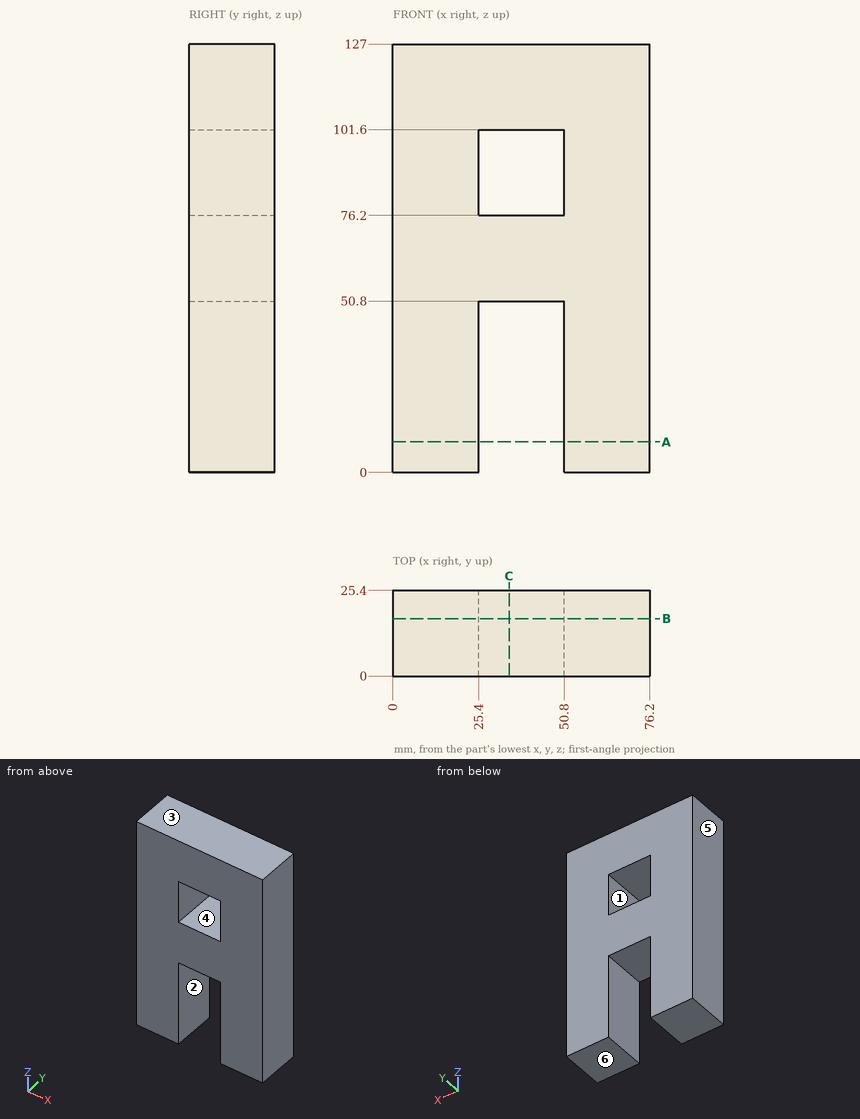
Part print with two shaded views. Sizes in mm from the minimum x, y, z corner. A direction names the side the tool comes from. Give positions to 0.01 mm unless a question says otherwise; leave off trailing zeros. Order: outer loops, then holes, each group sorted by start corner. A loop starts at its lowest first (then second) coordinate and runs counter-clockwise, first axis right, second up. Notation, with made-up numbers: M -12.5,0.5 L 13.5,0.5 A20 ccw 13.5,33.5 Z; hole C -11,42 d8. An arc over 180 degrees is marked long. Put each result on its own line as item: value.
Item 1: Cut at C-C on x = 34.5. Write the cut outline in (y, z), then the cut area to 3 significant figures.
Results are:
outline: M 0,50.8 L 25.4,50.8 L 25.4,76.2 L 0,76.2 Z; M 0,101.6 L 25.4,101.6 L 25.4,127 L 0,127 Z
area: 1,290 mm2
Item 2: Cut at B-B on y = 17. Write the cut outline in (x, z).
Results are:
outline: M 0,0 L 25.4,0 L 25.4,50.8 L 50.8,50.8 L 50.8,0 L 76.2,0 L 76.2,127 L 0,127 Z; hole M 25.4,76.2 L 50.8,76.2 L 50.8,101.6 L 25.4,101.6 Z
Item 3: Pull direction Z, two halves, no side cores. Call the marked faces 4, 5 and 6: +Z half, -Z half, draft (parallel to the pull), parting line (faces both ways), or undercut.
Results are:
face 4: undercut
face 5: draft
face 6: -Z half
Item 4: Cut at A-A on z = 9. Write the cut outline in (x, y), then the cut area to 3 significant figures.
Results are:
outline: M 0,0 L 25.4,0 L 25.4,25.4 L 0,25.4 Z; M 50.8,0 L 76.2,0 L 76.2,25.4 L 50.8,25.4 Z
area: 1,290 mm2
Item 5: Drop flat-ended pins along their axis: pin 1 Ø12 at (x, z) = (39.5, 95) entering from -Y; pin 2 Ø7.5 at (y, z) = (7.5, 85) entering from -X; pin 3 Ø5 at (x, y) = (34.5, 18.5) entering from -Z. Give the stop position or say it passes through.
Results are:
pin 1: through
pin 2: x = 0
pin 3: z = 50.8
Item 6: Which spindle directions (+Z, -Z, +X, -X, +Y, -Y) get a long thin tool onto all of the face, cutting with end or side? Do the marked faces 1, 2 and 3. Say none if no direction does.
Results are:
face 1: +Y, -Y
face 2: -Z, +Y, -Y
face 3: +Z, +X, -X, +Y, -Y
Item 7: Wall check: probe 1 along X at (y, z) = (21.75, 34); probe 2 along Z at (x, y) = (40, 21.25). Give the ranges that are in metal, low to high.
Results are:
probe 1: 0 to 25.4, 50.8 to 76.2
probe 2: 50.8 to 76.2, 101.6 to 127
